Model file for the job. Use its own axes, mm. Face numbers are marked on the shaded views. A direction names the side the tool comes from. Give positions to 0.01 mm unless a question says otherwise; leave off trailing zeros. Write each loop counter-clockwise with the first axis right and the second up, starting at its lowest first coordinate (ties: lowest second). Pieces come first, ordered by that corner, then holes. Notation, with made-up numbers: (19, -5) - (73, -5) arc R20 ccw to (73, 16) - close; hole circle Ø10 at (40, 5.5). An arc over 180 degrees is marked (long way). Use a Markdown table: item, result. Add a question column.
```python
from build123d import *

# Parameters (mm, degrees)
SKETCH1_R                = 5
BOSS_EXTRUDE1_DEPTH      = 5
BOSS_EXTRUDE1_DEPTH_BACK = 45
SKETCH2_W                = 10
SKETCH2_H                = 2.5
CUT_EXTRUDE1_DEPTH       = 6
CUT_EXTRUDE1_DEPTH_BACK  = 6


with BuildPart() as part:
    # Sketch1 → Boss-Extrude1 (new body, two sides)
    with BuildSketch(Plane(origin=(0, 0, 0), x_dir=(0, 0, -1), z_dir=(1, 0, 0))) as boss_extrude1_sk:
        Circle(SKETCH1_R)
    extrude(amount=BOSS_EXTRUDE1_DEPTH)
    extrude(boss_extrude1_sk.sketch, amount=-BOSS_EXTRUDE1_DEPTH_BACK)

    # Sketch2 → Cut-Extrude1 (cut, two sides)
    with BuildSketch(Plane(origin=(0, 0, 0), x_dir=(1, 0, 0), z_dir=(0, 1, 0))) as cut_extrude1_sk:
        with Locations((-40, -3.75)):
            Rectangle(SKETCH2_W, SKETCH2_H)
        with Locations((-40, 3.75)):
            Rectangle(SKETCH2_W, SKETCH2_H)
        with Locations((0, -3.75)):
            Rectangle(SKETCH2_W, SKETCH2_H)
        with Locations((0, 3.75)):
            Rectangle(SKETCH2_W, SKETCH2_H)
    extrude(amount=CUT_EXTRUDE1_DEPTH, mode=Mode.SUBTRACT)
    extrude(cut_extrude1_sk.sketch, amount=-CUT_EXTRUDE1_DEPTH_BACK, mode=Mode.SUBTRACT)


solid = part.part
```
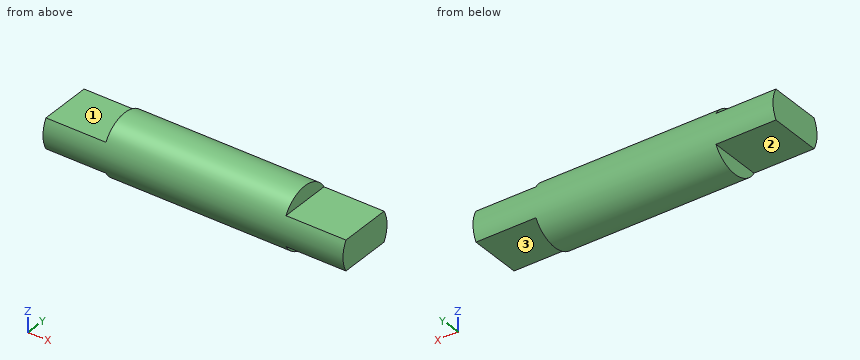
(1) Band-saw the part on A-A (y = -3). Write the cut outline in (x, z), then the cut area to 3 significant figures.
(2) Which spindle directions (+Z, -Z, +X, -X, +Y, -Y) get a long thin tool onto all of the face, cutting with end or side? Do the marked faces 1, 2 and 3. Say none if no direction does.
(3) Flat gauge pins, fed straight in: pin 1 (1.3 mm diameter, centred on y = 2, z = -3.5, fed in from +X); pin 2 (0.8 mm diameter, centred on y = 1.5, z = 4, fed in from -X); pin 3 (2 mm diameter, centred on x = -13.5, z = 3.5, fed in from +Y). Where does each tip first touch, or does it go through?
(4) Band-saw the part on C-C (x = -1). Write the cut outline in (y, z), then the cut area to 3 significant figures.
(5) Probe probe 1 along Z at (x, y) = (2.5, -1.5); probe 2 along Z at (x, y) = (-13.5, -0.25); probe 3 along X at (y, z) = (1, 3.25). List the from-to ranges inside material, lowest first. Write a range as [from, to].
(6) Band-saw the part on D-D (y = 0). Write the cut outline in (x, z), then the cut area to 3 significant figures.
(7) Band-saw the part on B-B (z = 4). Write the cut outline in (x, y), then the cut area to 3 significant figures.
Model answer:
| question | item | result |
|---|---|---|
| 1 | outline | (-45, -2.5) - (-35, -2.5) - (-35, -4) - (-5, -4) - (-5, -2.5) - (5, -2.5) - (5, 2.5) - (-5, 2.5) - (-5, 4) - (-35, 4) - (-35, 2.5) - (-45, 2.5) - close |
| 1 | area | 340 mm^2 |
| 2 | face 1 | +Z, -X, +Y, -Y |
| 2 | face 2 | -Z, -X, +Y, -Y |
| 2 | face 3 | -Z, +X, +Y, -Y |
| 3 | pin 1 | stops at x = -5 |
| 3 | pin 2 | stops at x = -35 |
| 3 | pin 3 | stops at y = 4.33 |
| 4 | outline | (-4.33, -2.5) - (4.33, -2.5) arc R5 ccw to (4.33, 2.5) - (-4.33, 2.5) arc R5 ccw to start |
| 4 | area | 47.8 mm^2 |
| 5 | probe 1 | z = [-2.5, 2.5] |
| 5 | probe 2 | z = [-4.99, 4.99] |
| 5 | probe 3 | x = [-35, -5] |
| 6 | outline | (-45, -2.5) - (-35, -2.5) - (-35, -5) - (-5, -5) - (-5, -2.5) - (5, -2.5) - (5, 2.5) - (-5, 2.5) - (-5, 5) - (-35, 5) - (-35, 2.5) - (-45, 2.5) - close |
| 6 | area | 400 mm^2 |
| 7 | outline | (-35, -3) - (-5, -3) - (-5, 3) - (-35, 3) - close |
| 7 | area | 180 mm^2 |
